CAD build for the part. Positions are in the model's coordinates, mm. A direction names the side the tool comes from. Round coordinates to 2 decimals unless told otherwise and drop trailing zeros. Loops run counter-clockwise (first coordinate to the right, second up) from the corner with the lowest first, then second, coordinate; pieces in that order, holes last.
```python
from build123d import *

# Parameters (mm, degrees)
F0_W      = 127
F0_H      = 127
F1_DEPTH  = 304.8
F2_W      = 101.6
F2_H      = 101.6
F3_DEPTH  = 292.1
F4_R      = 6.35
F5_DEPTH  = 127.001
F6_W      = 101.6
F6_H      = 101.6
F7_DEPTH  = 12.7
F8_W      = 127
F8_H      = 12.7
F9_DEPTH  = 330.2
F11_DEPTH = 127
F13_DEPTH = 127


with BuildPart() as f1:
    # F0 (on Top) → F1 (new body)
    with BuildSketch(Plane.XY):
        with Locations((3.740035, -2.651978)):
            Rectangle(F0_W, F0_H)
    extrude(amount=F1_DEPTH)

    # F2 (on face) → F3 (cut)
    with BuildSketch(Plane(origin=(0, 0, 0), x_dir=(1, 0, 0), z_dir=(0, 0, -1))):
        with Locations((3.740035, 2.651978)):
            Rectangle(F2_W, F2_H)
    extrude(amount=-F3_DEPTH, mode=Mode.SUBTRACT)

    # F4 (on face) → F5 (cut, through all)
    with BuildSketch(Plane(origin=(-59.759965, 0, 0), x_dir=(0, -1, 0), z_dir=(-1, 0, 0))):
        with Locations((2.651978, 190.5)):
            Circle(F4_R)
    extrude(amount=-F5_DEPTH, mode=Mode.SUBTRACT)

    # F6 (on face) → F7 (join)
    with BuildSketch(Plane(origin=(0, 0, 0), x_dir=(1, 0, 0), z_dir=(0, 0, -1))):
        with BuildLine():
            Line((3.740035, 66.151978), (302.190035, 66.151978))
            ThreePointArc((302.190035, 66.151978), (3.740035, 364.601978), (-294.709965, 66.151978))
            Line((-294.709965, 66.151978), (3.740035, 66.151978))
        make_face()
        with BuildLine():
            ThreePointArc((-294.709965, 66.151978), (3.740035, -232.298022), (302.190035, 66.151978))
            Line((302.190035, 66.151978), (3.740035, 66.151978))
            Line((3.740035, 66.151978), (-294.709965, 66.151978))
        make_face()
        with Locations((3.740035, 2.651978)):
            Rectangle(F6_W, F6_H, mode=Mode.SUBTRACT)
    extrude(amount=F7_DEPTH)

    # F8 (on face) → F9 (join)
    with BuildSketch(Plane.XY):
        with Locations((-123.259965, -204.855681)):
            Rectangle(F8_W, F8_H)
        with Locations((130.740035, -204.855681)):
            Rectangle(F8_W, F8_H)
    extrude(amount=F9_DEPTH)

    # F10 (on face) → F11 (join)
    with BuildSketch(Plane.YZ.offset(194.240035)):
        Polygon((-99.509686, 0), (-198.505681, 165.1), (-198.505681, 126.607434), (-122.590303, 0), align=None)
    extrude(amount=-F11_DEPTH)

    # F12 (on face) → F13 (join)
    with BuildSketch(Plane(origin=(-186.759965, 0, 0), x_dir=(0, -1, 0), z_dir=(-1, 0, 0))):
        Polygon((198.505681, 126.607495), (198.505681, 165.1), (99.509656, 0), (122.590244, 0), align=None)
    extrude(amount=-F13_DEPTH)


solid = f1.part
```
Item 1: Cut at C-C, the plane x = 173.5. Give the cut face in (y, z).
Answers follow:
outline: (-311.62, -12.7) - (179.31, -12.7) - (179.31, 0) - (-99.51, 0) - (-198.51, 165.1) - (-198.51, 330.2) - (-211.21, 330.2) - (-211.21, 0) - (-311.62, 0) - close; hole (-198.51, 0) - (-122.59, 0) - (-198.51, 126.61) - close
Item 2: 3-axis set-ups, long thin cutter, end or side, ignore diameter. For faces 1 (the flat face through (54.54, -2, 142)), 2 (the flat face through (-186.76, -180, 117)), 3 (the flat face through (131.63, -161.08, 64.19)), 4 (the flat face through (-124, -198.506, 246)), 5 (the flat face through (130, -211.206, 163)): which of +Z, -Z, +X, -X, +Y, -Y reach the whole face in a straight line?
Answers follow:
face 1: -Z
face 2: +Z, -X, +Y, -Y
face 3: +X, -X
face 4: +Z, +X, -X, +Y
face 5: +Z, +X, -X, -Y
Item 3: Probe line 1 (X direction, y = -15, z = 194.5); line 2 (Y direction, x = -76.5, z = 241.5); line 3 (Z direction, x = -132.5, y = 100). List the from-to ranges inside material, lowest first.
Answers follow:
line 1: x = -59.76 to -47.06, 54.54 to 67.24
line 2: y = -211.21 to -198.51
line 3: z = -12.7 to 0
Item 4: Cut at B-B, the plane x = -128. Give the cut face in (y, z).
Answers follow:
outline: (-333.95, -12.7) - (201.65, -12.7) - (201.65, 0) - (-99.51, 0) - (-198.51, 165.1) - (-198.51, 330.2) - (-211.21, 330.2) - (-211.21, 0) - (-333.95, 0) - close; hole (-198.51, 0) - (-122.59, 0) - (-198.51, 126.61) - close
Item 5: Two-plate mould, pull along X, no slides. Class faces 6 (the flat face through (3, -66.152, 150)), 7 (the flat face through (3, -53.452, 142)), 8 (the flat face through (-59.76, -4, 150)): released by +X, released by -X, zero draft, split by the parting line, or undercut.
Answers follow:
face 6: zero draft
face 7: undercut
face 8: released by -X
Item 6: Flat gauge pins, fed straight in: P1, Ø5, axis at x = -61.5, z = 188.5, coming from the -Y side; P2, Ø6, axis at x = -139, z = 256, coming from the +Y side; P3, Ø4, axis at x = 106, z = 44, coming from the +Y side. Where does each tip first touch, or does it go through?
Answers follow:
P1: stops at y = -211.21
P2: stops at y = -198.51
P3: stops at y = -124.69
Item 7: Cut at A-A, the plane z = 266. Give the cut face in (x, y), plus the area to 3 significant figures.
Answers follow:
outline: (-186.76, -211.21) - (-59.76, -211.21) - (-59.76, -198.51) - (-186.76, -198.51) - close; (-59.76, -66.15) - (67.24, -66.15) - (67.24, 60.85) - (-59.76, 60.85) - close; (67.24, -211.21) - (194.24, -211.21) - (194.24, -198.51) - (67.24, -198.51) - close; hole (-47.06, -53.45) - (54.54, -53.45) - (54.54, 48.15) - (-47.06, 48.15) - close
area: 9,030 mm2
Item 8: Cut at D-D, the plane y = -248.5. Give the cut face in (x, z), plus the area to 3 significant figures.
Answers follow:
outline: (-232.53, -12.7) - (240.01, -12.7) - (240.01, 0) - (-232.53, 0) - close
area: 6,000 mm2
